```python
from build123d import *

# Parameters (mm, degrees)
SKETCH1_W           = 120.2
SKETCH1_H           = 80.2
BOSS_EXTRUDE1_DEPTH = 1.6
SKETCH2_W           = 123.4
SKETCH2_H           = 83.4
SKETCH2_W_2         = 120.2
SKETCH2_H_2         = 80.2
BOSS_EXTRUDE2_DEPTH = 8.2
SKETCH3_W           = 120.2
SKETCH3_H           = 80.2
BOSS_EXTRUDE3_DEPTH = 5
SKETCH4_R           = 1.6
CUT_EXTRUDE1_DEPTH  = 5


with BuildPart() as part:
    # Sketch1 → Boss-Extrude1 (new body)
    with BuildSketch(Plane.XY):
        Rectangle(SKETCH1_W, SKETCH1_H)
    extrude(amount=BOSS_EXTRUDE1_DEPTH)

    # Sketch2 → Boss-Extrude2 (add)
    with BuildSketch(Plane.XY):
        Rectangle(SKETCH2_W, SKETCH2_H)
        Rectangle(SKETCH2_W_2, SKETCH2_H_2, mode=Mode.SUBTRACT)
    extrude(amount=BOSS_EXTRUDE2_DEPTH)

    # Sketch3 → Boss-Extrude3 (add)
    with BuildSketch(Plane.XY.offset(1.6)):
        Rectangle(SKETCH3_W, SKETCH3_H)
        Polygon((-58.5, 34.1), (-54.1, 34.1), (-54.1, 38.5), (54.1, 38.5), (54.1, 34.1), (58.5, 34.1), (58.5, -34.1), (54.1, -34.1), (54.1, -38.5), (-54.1, -38.5), (-54.1, -34.1), (-58.5, -34.1), align=None, mode=Mode.SUBTRACT)
    extrude(amount=BOSS_EXTRUDE3_DEPTH)

    # Sketch4 → Cut-Extrude1 (cut)
    with BuildSketch(Plane.XY.offset(6.6)):
        with Locations((-57, 37)):
            Circle(SKETCH4_R)
        with Locations((57, 37)):
            Circle(SKETCH4_R)
        with Locations((57, -37)):
            Circle(SKETCH4_R)
        with Locations((-57, -37)):
            Circle(SKETCH4_R)
    extrude(amount=-CUT_EXTRUDE1_DEPTH, mode=Mode.SUBTRACT)


solid = part.part
```
The model under review builds one solid part; all positions refer to its coordinate system, in mm. A direction names the side the tool comes from. Give positions to 0.01 mm unless a question says otherwise; leave off trailing zeros. Write each loop counter-clockwise with the first axis right and the second up, starting at its lowest first coordinate (ties: lowest second). Pieces come first, ordered by that corner, then holes. Notation, with made-up numbers: M 69.25,25.5 L 115.25,25.5 A32 ccw 115.25,58.5 Z; hole C -21.75,86 d11. An arc over 180 degrees is marked long. Write item = value, one per line. Start each with the question number.
Q1. We need section C-C (y = -8). State the section outline as (x, z) points, plus the area to 3 significant figures.
Q2. Machinability: for faces 1 (the face through (54.1, 36, 4)), 2 (the face through (61.7, -1, 4)), which of the approach directions +Z, -Z, +X, -X, +Y, -Y give a long, thin tool a straight path to every point of the face, cutting with its end or side? Answer none if there is none.
Q3. We need section A-A (z = 3). State the section outline as (x, y) points.
Q4. We need section D-D (x = -48.5). State the section outline as (y, z) points.
Q5. We need section B-B (x = 57). State the section outline as (y, z) points, plus the area to 3 significant figures.
Q6. For line 1 (Y direction, x = -57, z = 4.9); line 2 (Y direction, x = 20.5, z = 5.25); line 3 (X direction, y = 13, z = 1.75), list the stretches that pass through material, from the lowest coordinate up.
Q7. Clearance check with a flat-ended pin moving along its axis: pin 1 (8 mm diameter, centred on x = -15.5, y = 32.5, fed in from +Z). State where the tip first meets the part, or that it passes through.
Result set:
q1.outline = M -61.7,0 L 61.7,0 L 61.7,8.2 L 60.1,8.2 L 60.1,6.6 L 58.5,6.6 L 58.5,1.6 L -58.5,1.6 L -58.5,6.6 L -60.1,6.6 L -60.1,8.2 L -61.7,8.2 Z
q1.area = 235 mm2
q2.face_1 = +Z
q2.face_2 = +Z, -Z, +X, +Y, -Y
q3.outline = M -61.7,-41.7 L 61.7,-41.7 L 61.7,41.7 L -61.7,41.7 Z; hole C -57,-37 d3.2; hole C -57,37 d3.2; hole M -58.5,-34.1 L -54.1,-34.1 L -54.1,-38.5 L 54.1,-38.5 L 54.1,-34.1 L 58.5,-34.1 L 58.5,34.1 L 54.1,34.1 L 54.1,38.5 L -54.1,38.5 L -54.1,34.1 L -58.5,34.1 Z; hole C 57,-37 d3.2; hole C 57,37 d3.2
q4.outline = M -41.7,0 L 41.7,0 L 41.7,8.2 L 40.1,8.2 L 40.1,6.6 L 38.5,6.6 L 38.5,1.6 L -38.5,1.6 L -38.5,6.6 L -40.1,6.6 L -40.1,8.2 L -41.7,8.2 Z
q5.outline = M -41.7,0 L 41.7,0 L 41.7,8.2 L 40.1,8.2 L 40.1,6.6 L 38.6,6.6 L 38.6,1.6 L 35.4,1.6 L 35.4,6.6 L 34.1,6.6 L 34.1,1.6 L -34.1,1.6 L -34.1,6.6 L -35.4,6.6 L -35.4,1.6 L -38.6,1.6 L -38.6,6.6 L -40.1,6.6 L -40.1,8.2 L -41.7,8.2 Z
q5.area = 183 mm2
q6.line_1 = -41.7 to -38.6, -35.4 to -34.1, 34.1 to 35.4, 38.6 to 41.7
q6.line_2 = -41.7 to -38.5, 38.5 to 41.7
q6.line_3 = -61.7 to -58.5, 58.5 to 61.7
q7.pin_1 = 1.6
